```python
from build123d import *

# Parameters (mm, degrees)
SKETCH1_R                = 9
BRACKETMOUNT_DEPTH       = 5
SKETCH2_R                = 1
BRACKET_MOUNTHOLES_DEPTH = 5
SKETCH3_R                = 4
STEPPERSLEEVE_DEPTH      = 1094
ORIENTATIONNUB_DEPTH     = 1094


with BuildPart() as part:
    # Sketch1 → BracketMount (new body)
    with BuildSketch(Plane(origin=(0, 0, 0), x_dir=(1, 0, 0), z_dir=(0, 1, 0))):
        with Locations(Location((0, 0, 0), (0, 0, 270))):
            Circle(SKETCH1_R)
    extrude(amount=BRACKETMOUNT_DEPTH)

    # Sketch2 → Bracket-MountHoles (cut)
    with BuildSketch(Plane(origin=(0, 5, 0), x_dir=(1, 0, 0), z_dir=(0, 1, 0))):
        with Locations(Location((0, 7.25, 0), (0, 0, 270))):
            Circle(SKETCH2_R)
        with Locations(Location((7.25, 0, 0), (0, 0, 270))):
            Circle(SKETCH2_R)
        with Locations(Location((0, -7.25, 0), (0, 0, 270))):
            Circle(SKETCH2_R)
        with Locations(Location((-7.25, 0, 0), (0, 0, 270))):
            Circle(SKETCH2_R)
    extrude(amount=-BRACKET_MOUNTHOLES_DEPTH, mode=Mode.SUBTRACT)

    # Sketch3 → StepperSleeve (add)
    with BuildSketch(Plane.XZ):
        with Locations(Location((0, 0, 0), (0, 0, 90))):
            Circle(SKETCH3_R)
    extrude(amount=STEPPERSLEEVE_DEPTH)

    # Sketch5 → OrientationNub (cut)
    with BuildSketch(Plane.XZ.offset(1094)):
        with BuildLine():
            Line((1.92, 1.75316856), (1.92, -1.75316856))
            ThreePointArc((1.92, -1.75316856), (-2.6, 0), (1.92, 1.75316856))
        make_face()
    extrude(amount=-ORIENTATIONNUB_DEPTH, mode=Mode.SUBTRACT)


solid = part.part
```
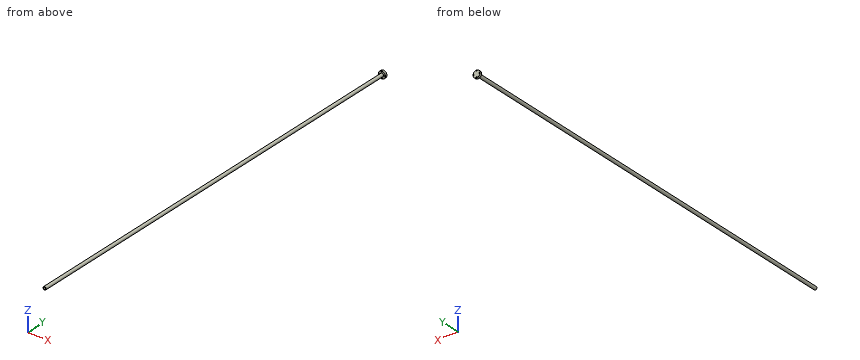
Can you work these out from the model? Positions are in its coordinate system, mm. Round coordinates to 2 decimals unless told otherwise and drop trailing zeros. Order: outer loops, then holes, each group sorted by start corner. A loop starts at its lowest first (then second) coordinate and runs counter-clockwise, first axis right, second up.
(1) If I drill on L1, parallel to X at y = 3.6, z = 0; L2, parallel to Z at x = 0.25, y = -371; L3, parallel to Y at x = -3.5, z = -6, over which ranges is the centre line in solid material (lowest first)?
Results are:
L1: x = -9 to -8.25, -6.25 to 6.25, 8.25 to 9
L2: z = -3.99 to -2.59, 2.59 to 3.99
L3: y = 0 to 5
(2) If we section it at A-A (y = -777): Please give me the cut outline in (x, z), plus the area to 3 significant figures.
Results are:
outline: circle Ø8 at (0, 0); hole (1.92, -1.75) - (1.92, 1.75) arc R2.6 ccw (long way) to start
area: 30.7 mm2
(3) I'm going to push flat-ended pins straight in: pin 1 (1.2 mm diameter, centred on x = 0, z = -7.25, fed in from -Y); pin 2 (6 mm diameter, centred on y = -396, z = 2, fed in from -X); pin 3 (2.5 mm diameter, centred on x = -7.25, z = 0, fed in from -Y); pin 4 (5.5 mm diameter, centred on x = -0.5, z = 1, fed in from -Y). Where does each tip first touch, or does it pass through?
Results are:
pin 1: passes through
pin 2: stops at x = -4
pin 3: stops at y = 0
pin 4: stops at y = -1094
